Could you check a few things on this model? Use its own coordinates, in mm. Face numbers are marked on the shaded views. A direction names the side the tool comes from. Give positions to 0.01 mm unless a question says otherwise; leave off trailing zeros. Loops run counter-clockwise (first coordinate to the right, second up) from the corner with the lowest first, then second, coordinate; pieces in that order, holes last.
1. Imagine slicing it at C-C (z = -19). List the corners of the cut face in (x, y) for me.
2. Imagine slicing it at A-A (z = -2.75). List the corners of the cut face in (x, y) for me.
3. Imagine slicing it at B-B (x = 0). List the corners of the cut face in (y, z) for me, plus the area to 3 significant figures.
4. Thinking about a two-plate mould opening in Y: for the marked faces 3, 4 and 5, which applies, +Y half, -Y half, draft (parallel to the pull), parting line (faces both ways), or undercut?
5. I need wall thicknesses on line 1 along Y through (x, z) = (0, -0.75); line 2 along Z through (x, y) = (-1.5, -0.1); line 3 along Z through (x, y) = (0.65, -0.4). Which ranges of each line are inside material? Lowest first, please.
6. For the marked faces 1 and 2, which set-ups out of +Z, -Z, +X, -X, +Y, -Y let a thin tool reach every point of the face, with its end or its side?
7. For P1, Ø2, axis at x = 0, y = 0, coming from the +Z side; P2, Ø1, axis at y = -1, z = -22.5, coming from the -X side, each with a flat end and sliding along its axis, tell me the tip position at first contact or that it passes through.
Autodesk Inventor part; units mm, degrees
ref_plane "YZ Plane" through (0, 0, 0) normal (1, 0, 0) x (0, 1, 0)
ref_plane "XZ Plane" through (0, 0, 0) normal (0, 1, 0) x (-1, 0, 0)
ref_plane "XY Plane" through (0, 0, 0) normal (0, 0, 1) x (1, 0, 0)
sketch "Sketch1" plane through (0, 0, 0) normal (0, 0, 1) x (1, 0, 0)
  line L0 (1.4434, -2.5) -> (-1.4434, -2.5)
  line L1 (-1.4434, -2.5) -> (-2.8868, 0)
  line L2 (-2.8868, 0) -> (-1.4434, 2.5)
  line L3 (-1.4434, 2.5) -> (1.4434, 2.5)
  line L4 (1.4434, 2.5) -> (2.8868, 0)
  line L5 (2.8868, 0) -> (1.4434, -2.5)
  point P0 (0, 0)
  point P1 (0, 0)
  dimension "d0" = 5
extrude "Extrusion1" add sketch "Sketch1" against normal blind 20
sketch "Sketch2" plane through (0, 0, 0) normal (0, 0, 1) x (1, 0, 0)
  circle A0 centre (0, 0) radius 1.25
  dimension "d3" = 2.5
extrude "Extrusion2" cut sketch "Sketch2" against normal blind 3
sketch "Sketch3" plane through (0, 0, -20) normal (0, 0, -1) x (-1, 0, 0)
  circle A0 centre (0, 0) radius 1.25
  dimension "d6" = 2.5
extrude "Extrusion3" add sketch "Sketch3" along normal blind 6
thread "Thread1"
thread "Thread2"
fillet "Fillet1" radius 0.2 12 edges at (0, -2.5, -20) (-2.1651, -1.25, -20) (-2.1651, 1.25, -20) (0, 2.5, -20) (2.1651, 1.25, -20) (2.1651, -1.25, -20) (0, -2.5, 0) (2.1651, -1.25, 0) (2.1651, 1.25, 0) (0, 2.5, 0) (-2.1651, 1.25, 0) (-2.1651, -1.25, 0)
fillet "Fillet1" radius 0.2 6 edges at (-2.8868, 0, -10) (-1.4434, 2.5, -10) (1.4434, 2.5, -10) (2.8868, 0, -10) (1.4434, -2.5, -10) (-1.4434, -2.5, -10)
sketch "Sketch4" plane through (0, 0, 0) normal (0, 0, 1) x (1, 0, 0)
  point P0 (0, 0)
equation "\"d0\" = m3hs_hexDiam"
equation "\"d3\" = m3hs_threadDiam"
equation "\"d4\" = m3hs_holeDepth"
equation "\"d6\" = m3hs_threadDiam"
equation "\"d7\" = m3hs_studLength"
equation "\"d13\" = m3hs_rounding"
equation "\"m3hs_hexDiam\" = 5"
equation "\"m3hs_bodyLength\" = 5"
equation "\"m3hs_holeDepth\" = 3"
equation "\"m3hs_studLength\" = 6"
equation "\"m3hs_rounding\" = 0.2"
equation "\"m3hs_threadDiam\" = 2.5"
properties part number "M2.5 Hex Spacer 5mm" material "Stainless Steel"
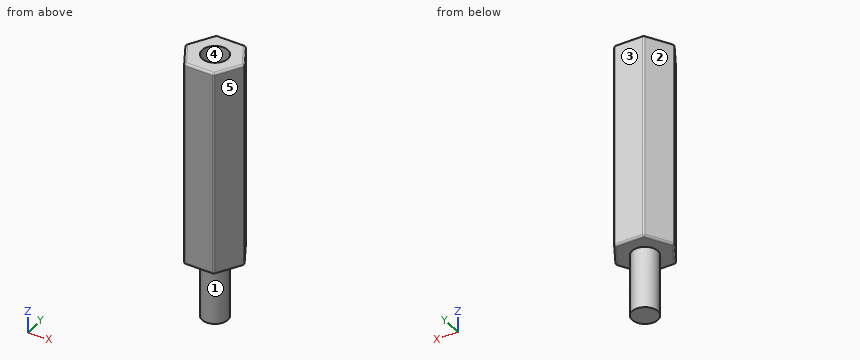
Derived:
1. outline: (-2.83, -0.1) - (-1.5, -2.4) arc R0.2 ccw to (-1.33, -2.5) - (1.33, -2.5) arc R0.2 ccw to (1.5, -2.4) - (2.83, -0.1) arc R0.2 ccw to (2.83, 0.1) - (1.5, 2.4) arc R0.2 ccw to (1.33, 2.5) - (-1.33, 2.5) arc R0.2 ccw to (-1.5, 2.4) - (-2.83, 0.1) arc R0.2 ccw to start
2. outline: (-2.83, -0.1) - (-1.5, -2.4) arc R0.2 ccw to (-1.33, -2.5) - (1.33, -2.5) arc R0.2 ccw to (1.5, -2.4) - (2.83, -0.1) arc R0.2 ccw to (2.83, 0.1) - (1.5, 2.4) arc R0.2 ccw to (1.33, 2.5) - (-1.33, 2.5) arc R0.2 ccw to (-1.5, 2.4) - (-2.83, 0.1) arc R0.2 ccw to start; hole circle Ø2.5 at (0, 0)
3. outline: (-2.5, -19.8) arc R0.2 ccw to (-2.3, -20) - (-1.25, -20) - (-1.25, -26) - (1.25, -26) - (1.25, -20) - (2.3, -20) arc R0.2 ccw to (2.5, -19.8) - (2.5, -0.2) arc R0.2 ccw to (2.3, 0) - (1.25, 0) - (1.25, -3) - (-1.25, -3) - (-1.25, 0) - (-2.3, 0) arc R0.2 ccw to (-2.5, -0.2) - close
3. area: 107 mm2
4. face 3: +Y half
4. face 4: undercut
4. face 5: -Y half
5. line 1: y = -2.5 to -1.25, 1.25 to 2.5
5. line 2: z = -20 to 0
5. line 3: z = -26 to -3
6. face 1: -Z
6. face 2: +Z, -Z, -X, +Y
7. P1: stops at z = -3
7. P2: stops at x = -1.15
